Geometry: see drawing. Coordinates: mm, zero at the bounding-box minimum. A direction names the side the tool comes from. Round coordinates to 2 decimals unless told otherwise and drop trailing zeros. Order: outer loops, then holes, each group sorted by start corner. A loop starts at its lowest first (then second) coordinate and runs counter-clockwise, first axis right, second up. Notation, with made-up numbers: (46.5, 35.25) - (56.5, 35.25) arc R24 cw to (56.5, 51.25) - close; hole circle Ø7 at (84, 41). An arc over 180 degrees is marked (long way). Put each result on its own line as item: value. Start each with the question number.
1) Section B-B on y = 20.5. Output: boundary loops of the cut face in (x, z).
2) Section A-A on x = 7. Output: boundary loops of the cut face in (y, z).
3) Access query for the marked faces 1, 2 and 3. Directions: +Z, -Z, +X, -X, +Y, -Y. A direction counts if a zero-diameter tool reaches every point of the face in a straight line with its end or side. Return the directions, or none.
4) Section D-D on x = 14.5. Output: boundary loops of the cut face in (y, z).
5) Section C-C on z = 0.5. Output: boundary loops of the cut face in (x, y).
6) Line query: probe 1 along Y at (x, z) = (6.75, 3.3); probe 2 along Z at (x, y) = (24.5, 48); probe 3 along Y at (x, z) = (20, 1.9). Output: solid intervals per line, ascending. Write a range as [from, to].
7) Contact query for flat-ended pins moving along their axis: P1, Ø0.8, axis at y = 50, z = 1.5, coming from the -X side; P2, Ø4, axis at x = 8, y = 45.5, coming from the +Z side; P3, Ø1, axis at x = 7, z = 1, coming from the -Y side. Output: stop coordinate, or through.
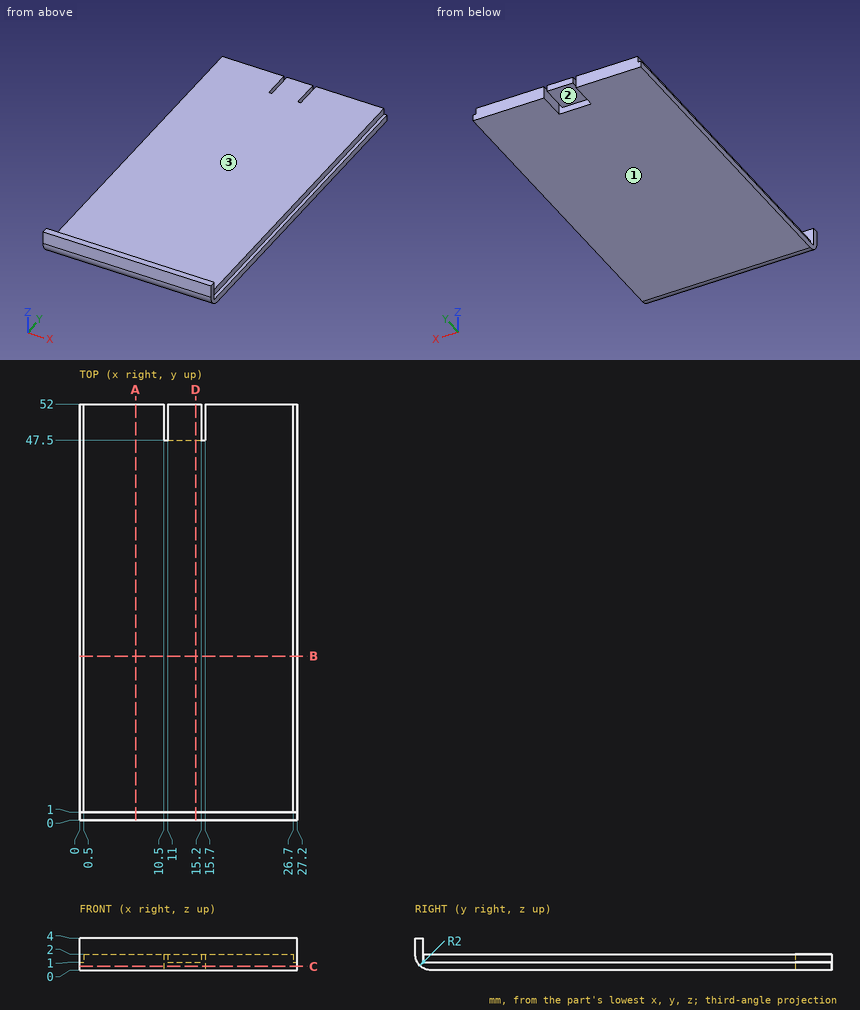
Answer sheet:
1. outline: (0, 0) - (27.2, 0) - (27.2, 1) - (26.7, 1) - (26.7, 2) - (0.5, 2) - (0.5, 1) - (0, 1) - close
2. outline: (0, 2) arc R2 ccw to (2, 0) - (52, 0) - (52, 2) - (1, 2) - (1, 4) - (0, 4) - close
3. face 1: -Z, +X, -X, +Y, -Y
3. face 2: -Z, +Y
3. face 3: +Z, +X, -X, +Y
4. outline: (0, 2) arc R2 ccw to (2, 0) - (47.5, 0) - (47.5, 1) - (52, 1) - (52, 2) - (1, 2) - (1, 4) - (0, 4) - close
5. outline: (0, 0.68) - (27.2, 0.68) - (27.2, 52) - (15.7, 52) - (15.7, 47.5) - (10.5, 47.5) - (10.5, 52) - (0, 52) - close
6. probe 1: [0, 1]
6. probe 2: [0, 2]
6. probe 3: [0, 52]
7. P1: x = 0.5
7. P2: z = 2
7. P3: y = 0.06
